Build history of the part. All positions in model axes, mm. A direction names the side the tool comes from. Coordinates: 2 decimals unless noted, no trailing zeros. Order: outer loops, then holes, each group sorted by start corner. A loop starts at its lowest first (then second) coordinate and runs counter-clockwise, first axis right, second up. Notation, with made-up numbers: (38, 9) - (80, 9) arc R9 ccw to (80, 21) - close; hole circle Ø8 at (18, 80). An arc over 180 degrees is marked (long way). Write each question's results on one line, items separated by ' | '.
from build123d import *

# Parameters (mm, degrees)
SKETCH4_W           = 54
SKETCH4_H           = 42
BOSS_EXTRUDE1_DEPTH = 5
SKETCH5_R           = 6
SKETCH5_R_2         = 3
CUT_EXTRUDE1_DEPTH  = 5
SKETCH6_W           = 7.5
SKETCH6_H           = 7.5
BOSS_EXTRUDE3_DEPTH = 20


with BuildPart() as part:
    # Sketch4 → Boss-Extrude1 (new body)
    with BuildSketch(Plane(origin=(0, 0, 0), x_dir=(1, 0, 0), z_dir=(0, 1, 0))):
        Rectangle(SKETCH4_W, SKETCH4_H)
    extrude(amount=BOSS_EXTRUDE1_DEPTH)

    # Sketch5 → Cut-Extrude1 (cut)
    with BuildSketch(Plane(origin=(0, 5, 0), x_dir=(1, 0, 0), z_dir=(0, 1, 0))):
        with Locations(Location((0, 0, 0), (0, 0, 270))):
            Circle(SKETCH5_R)
        with Locations(Location((-16, 0, 0), (0, 0, 270))):
            Circle(SKETCH5_R_2)
        with Locations(Location((16, 0, 0), (0, 0, 270))):
            Circle(SKETCH5_R_2)
    extrude(amount=-CUT_EXTRUDE1_DEPTH, mode=Mode.SUBTRACT)

    # Sketch6 → Boss-Extrude3 (add)
    with BuildSketch(Plane(origin=(0, 5, 0), x_dir=(1, 0, 0), z_dir=(0, 1, 0))):
        with Locations((-18.25, 12.25)):
            Rectangle(SKETCH6_W, SKETCH6_H)
        with Locations((18.25, 12.25)):
            Rectangle(SKETCH6_W, SKETCH6_H)
        with Locations((-18.25, -12.25)):
            Rectangle(SKETCH6_W, SKETCH6_H)
        with Locations((18.25, -12.25)):
            Rectangle(SKETCH6_W, SKETCH6_H)
    extrude(amount=BOSS_EXTRUDE3_DEPTH)


solid = part.part
1. Band-saw the part on C-C on z = 0. Give the cut face in (x, y).
Solved:
outline: (-27, 0) - (-19, 0) - (-19, 5) - (-27, 5) - close; (-13, 0) - (-6, 0) - (-6, 5) - (-13, 5) - close; (6, 0) - (13, 0) - (13, 5) - (6, 5) - close; (19, 0) - (27, 0) - (27, 5) - (19, 5) - close
2. Band-saw the part on A-A on x = 0. Give the cut face in (y, z).
Solved:
outline: (0, -21) - (5, -21) - (5, -6) - (0, -6) - close; (0, 6) - (5, 6) - (5, 21) - (0, 21) - close
3. Band-saw the part on B-B on y = 17.25. Give the cut face in (x, z), then the cut area to 3 significant figures.
Solved:
outline: (-22, -16) - (-14.5, -16) - (-14.5, -8.5) - (-22, -8.5) - close; (-22, 8.5) - (-14.5, 8.5) - (-14.5, 16) - (-22, 16) - close; (14.5, -16) - (22, -16) - (22, -8.5) - (14.5, -8.5) - close; (14.5, 8.5) - (22, 8.5) - (22, 16) - (14.5, 16) - close | area: 225 mm2
4. Drop flat-ended pins along their axis: pin 1 Ø8 at (y, z) = (18.5, -13.5) entering from -X; pin 2 Ø9.5 at (x, z) = (-16, 0) entering from +Y; pin 3 Ø6 at (x, y) = (18, 17) entering from -Z; pin 4 Ø1.5 at (y, z) = (13, -6) entering from -X. Give the stop position or say it passes through.
Solved:
pin 1: stops at x = -22 | pin 2: stops at y = 5 | pin 3: stops at z = -16 | pin 4: passes through
5. Two-plate mould, pull along Z, no slides. Class faces 1 (the face through (18, 15, -16)), 2 (the face through (14.5, 15, 12)), 3 (the face through (18, 15, 8.5)): +Z half, -Z half, draft (parallel to the pull), parting line (faces both ways), or undercut.
Solved:
face 1: -Z half | face 2: draft | face 3: undercut
6. Probe line 1 (X direction, y = 2.3, z = 0); line 2 (Z direction, x = -16, y = 21); line 3 (X direction, y = 13.5, z = -15.5). List the from-to ranges inside material, lowest first.
Solved:
line 1: x = -27 to -19, -13 to -6, 6 to 13, 19 to 27 | line 2: z = -16 to -8.5, 8.5 to 16 | line 3: x = -22 to -14.5, 14.5 to 22
7. Tool access for faces 4 (the face through (-14.5, 15, 12)), 5 (the face through (-18, 15, -16)), 6 (the face through (-18, 15, 8.5)), 7 (the face through (22, 15, 12)), 8 (the face through (-22, 15, 12)): list every direction of +Z, -Z, +X, -X, +Y, -Y with a clear straight run to the whole face (end or side of a thin tool).
Solved:
face 4: +Z, -Z, +Y | face 5: -Z, +X, -X, +Y | face 6: +X, -X, +Y | face 7: +Z, -Z, +X, +Y | face 8: +Z, -Z, -X, +Y
8. Band-saw the part on D-D on y = 3.5. Give the cut face in (x, z), then the cut area to 3 significant figures.
Solved:
outline: (-27, -21) - (27, -21) - (27, 21) - (-27, 21) - close; hole circle Ø6 at (-16, 0); hole circle Ø12 at (0, 0); hole circle Ø6 at (16, 0) | area: 2,100 mm2
